Design review of the part built by this model. Coordinates are the model's own, in mm. Coordinates: 2 decimals unless noted, no trailing zeros. Order: outer loops, then holes, each group sorted by start corner. A loop starts at its lowest first (then second) coordinate and runs counter-clockwise, first axis right, second up. Notation, with made-up numbers: M 55.5,45.5 L 84.5,45.5 A20 cw 84.5,57.5 Z; hole C -19.5,42 d8. An arc over 180 degrees is marked long. Use CSV: the item, a comma, the result in double quotes.
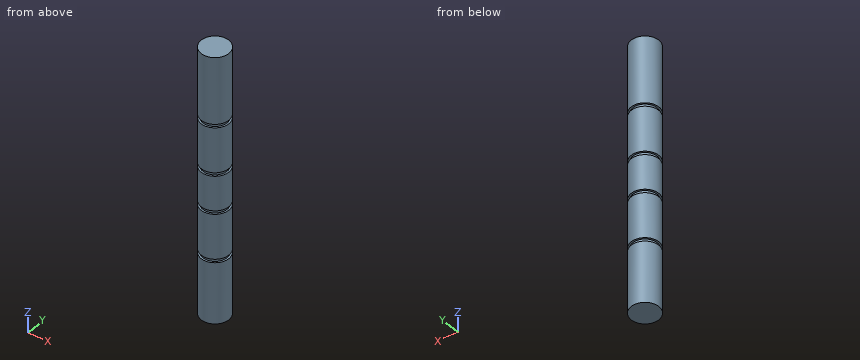
```python
from build123d import *

# Parameters (mm, degrees)
SKETCH1_R           = 3.5
BOSS_EXTRUDE1_DEPTH = 77
SKETCH3_R           = 4
SKETCH3_R_2         = 3.5
BOSS_EXTRUDE2_DEPTH = 17.7
SKETCH6_R           = 4
SKETCH6_R_2         = 3
BOSS_EXTRUDE3_DEPTH = 13
SKETCH7_R           = 4
SKETCH7_R_2         = 3
BOSS_EXTRUDE4_DEPTH = 10
SKETCH8_R           = 4
SKETCH8_R_2         = 3
BOSS_EXTRUDE5_DEPTH = 13
SKETCH9_R           = 4
SKETCH9_R_2         = 3
BOSS_EXTRUDE6_DEPTH = 19.3


with BuildPart() as part:
    # Sketch1 → Boss-Extrude1 (new body)
    with BuildSketch(Plane.XY):
        Circle(SKETCH1_R)
    extrude(amount=BOSS_EXTRUDE1_DEPTH)

    # Sketch3 → Boss-Extrude2 (add)
    with BuildSketch(Plane(origin=(0, 0, 0), x_dir=(-1, 0, 0), z_dir=(0, 0, -1))):
        Circle(SKETCH3_R)
        Circle(SKETCH3_R_2, mode=Mode.SUBTRACT)
    extrude(amount=-BOSS_EXTRUDE2_DEPTH)

    # Sketch6 → Boss-Extrude3 (add)
    with BuildSketch(Plane.XY.offset(18.7)):
        with Locations(Location((0, 0, 0), (0, 0, 180))):
            Circle(SKETCH6_R)
        Circle(SKETCH6_R_2, mode=Mode.SUBTRACT)
    extrude(amount=BOSS_EXTRUDE3_DEPTH)

    # Sketch7 → Boss-Extrude4 (add)
    with BuildSketch(Plane.XY.offset(32.7)):
        with Locations(Location((0, 0, 0), (0, 0, 180))):
            Circle(SKETCH7_R)
        Circle(SKETCH7_R_2, mode=Mode.SUBTRACT)
    extrude(amount=BOSS_EXTRUDE4_DEPTH)

    # Sketch8 → Boss-Extrude5 (add)
    with BuildSketch(Plane.XY.offset(43.7)):
        with Locations(Location((0, 0, 0), (0, 0, 180))):
            Circle(SKETCH8_R)
        Circle(SKETCH8_R_2, mode=Mode.SUBTRACT)
    extrude(amount=BOSS_EXTRUDE5_DEPTH)

    # Sketch9 → Boss-Extrude6 (add)
    with BuildSketch(Plane.XY.offset(57.7)):
        with Locations(Location((0, 0, 0), (0, 0, 180))):
            Circle(SKETCH9_R)
        Circle(SKETCH9_R_2, mode=Mode.SUBTRACT)
    extrude(amount=BOSS_EXTRUDE6_DEPTH)


solid = part.part
```
(1) Wall thickness on probe 1 along Z at (x, y) = (2, 3); probe 2 along Y at (x, z) = (-0.25, 25); probe 3 along Y at (x, z) = (-2, 9.5): over which ranges is each line inside the solid? List them lowest first.
The answers:
probe 1,"z = 0 to 17.7, 18.7 to 31.7, 32.7 to 42.7, 43.7 to 56.7, 57.7 to 77"
probe 2,"y = -3.99 to 3.99"
probe 3,"y = -3.46 to 3.46"
(2) Add section A-A on z = 26.5. State the section outline as (x, y) points, and give its area (3 significant figures).
The answers:
outline,"C 0,0 d8"
area,"50.3 mm2"
(3) Clearance check with flat-ended pins moving along their axes: P1, Ø4, axis at x = 2.5, z = 43.5, coming from the -Y side; P2, Ø1.5, axis at x = 1, z = 32.5, coming from the +Y side; P3, Ø4, axis at y = -2, z = 60.5, coming from the +X side; P4, Ø1, axis at x = 2.5, z = 8.5, coming from the +Y side. State where each tip first meets the part, or that it passes through.
The answers:
P1,"stops at y = -3.97"
P2,"stops at y = 3.99"
P3,"stops at x = 4"
P4,"stops at y = 3.46"
